from build123d import *

# Parameters (mm, degrees)
SKETCH1_W           = 19.05
SKETCH1_H           = 19.05
SKETCH1_W_2         = 14.2875
SKETCH1_H_2         = 14.2875
BOSS_EXTRUDE1_DEPTH = 25.4
CUT_EXTRUDE1_REACH  = 21.05
SKETCH2_R           = 3.175
SKETCH3_R           = 4
BOSS_EXTRUDE2_DEPTH = 31.75
FILLET1_R           = 2.54


with BuildPart() as part:
    # Sketch1 → Boss-Extrude1 (new body)
    with BuildSketch(Plane(origin=(0, 0, 0), x_dir=(1, 0, 0), z_dir=(0, 1, 0))):
        with Locations((9.525, 9.525)):
            Rectangle(SKETCH1_W, SKETCH1_H)
        with Locations((9.525, 9.525)):
            Rectangle(SKETCH1_W_2, SKETCH1_H_2, mode=Mode.SUBTRACT)
    extrude(amount=BOSS_EXTRUDE1_DEPTH)

    # Sketch2 → Cut-Extrude1 (cut, up to next)
    with BuildSketch(Plane.XY, mode=Mode.PRIVATE) as cut_extrude1_sk1:
        with Locations((9.525, 12.7)):
            Circle(SKETCH2_R)
    cut_extrude1_tool1 = extrude(cut_extrude1_sk1.sketch, amount=-CUT_EXTRUDE1_REACH, mode=Mode.PRIVATE) & part.part
    add(cut_extrude1_tool1.solids().sort_by_distance((9.525, 12.7, 0))[0], mode=Mode.SUBTRACT)

    # Sketch3 → Boss-Extrude2 (add)
    with BuildSketch(Plane(origin=(19.05, 0, 0), x_dir=(0, 0, -1), z_dir=(1, 0, 0))):
        with Locations((9.525, 12.7)):
            Circle(SKETCH3_R)
    extrude(amount=BOSS_EXTRUDE2_DEPTH)

    # Fillet1
    fillet1_edges = [part.edges().sort_by_distance(p)[0] for p in [
        (2.38125, 12.7, -16.66875),
        (2.38125, 12.7, -2.38125),
        (16.66875, 12.7, -2.38125),
        (16.66875, 12.7, -16.66875),
        (0, 12.7, -19.05),
        (19.05, 12.7, -19.05),
        (19.05, 12.7, 0),
        (0, 12.7, 0),
    ]]
    fillet(fillet1_edges, radius=FILLET1_R)


solid = part.part
Input: part model. Units: mm. Frame: model coordinates. A direction names the side the tool comes from. Give positions to 0.01 mm unless a question says otherwise; leave off trailing zeros. Order: outer loops, then holes, each group sorted by start corner. A loop starts at its lowest first (then second) coordinate and runs counter-clockwise, first axis right, second up. Notation, with made-up numbers: (9.5, -9.5) - (47.5, -9.5) arc R16 ccw to (47.5, 18.5) - close; hole circle Ø5 at (29.25, 18). An arc over 180 degrees is marked (long way). Write each question's results on one line, items separated by ' | '.
Item 1: Section C-C (y = 12.7). Return loops of the section in (x, z) (3 decimals).
A:
outline: (0, -16.51) arc R2.54 ccw to (2.54, -19.05) - (16.51, -19.05) arc R2.54 ccw to (19.05, -16.51) - (19.05, -13.525) - (50.8, -13.525) - (50.8, -5.525) - (19.05, -5.525) - (19.05, -2.54) arc R2.54 ccw to (16.51, 0) - (12.7, 0) - (12.7, -2.381) - (14.129, -2.381) arc R2.54 cw to (16.669, -4.921) - (16.669, -14.129) arc R2.54 cw to (14.129, -16.669) - (4.921, -16.669) arc R2.54 cw to (2.381, -14.129) - (2.381, -4.921) arc R2.54 cw to (4.921, -2.381) - (6.35, -2.381) - (6.35, 0) - (2.54, 0) arc R2.54 ccw to (0, -2.54) - close
Item 2: Contact query for flat-ended pins moving along their axis: pin 1 Ø4 at (x, z) = (27.5, -10.5) entering from +Y; pin 2 Ø12 at (x, y) = (45.5, 22) entering from +Z; pin 3 Ø2 at (y, z) = (7, -4) entering from +X. Output: stop coordinate, or through.
A:
pin 1: stops at y = 16.7 | pin 2: stops at z = -7.26 | pin 3: stops at x = 19.05
Item 3: Section D-D (x = 30). Return loops of the section in (y, z) (3 decimals), and give its area (3 significant figures).
A:
outline: circle Ø8 at (12.7, -9.525) | area: 50.3 mm^2
Item 4: Access query for faces 5 (the cylindrical face through (34.7, 9.15, -11.37)), 6 (the cylindrical face through (18.286, 12.878, -0.724)), 7 (the cylindrical face through (3.145, 12.878, -3.106)). Directions: +Z, -Z, +X, -X, +Y, -Y. A direction counts if a zero-diameter tool reaches every point of the face in a straight line with its end or side. Return the directions, or none.
A:
face 5: +X | face 6: +Z, +X, +Y, -Y | face 7: +Y, -Y
Item 5: Section B-B (z = -15.5). Return loops of the section in (x, y).
A:
outline: (0, 0) - (2.78, 0) - (2.78, 25.4) - (0, 25.4) - close; (16.27, 0) - (19.05, 0) - (19.05, 25.4) - (16.27, 25.4) - close
Item 6: Section A-A (y = 3.75). Return loops of the section in (x, z), and give its area (3 significant figures).
A:
outline: (0, -16.51) arc R2.54 ccw to (2.54, -19.05) - (16.51, -19.05) arc R2.54 ccw to (19.05, -16.51) - (19.05, -2.54) arc R2.54 ccw to (16.51, 0) - (2.54, 0) arc R2.54 ccw to (0, -2.54) - close; hole (2.38, -14.13) arc R2.54 ccw to (4.92, -16.67) - (14.13, -16.67) arc R2.54 ccw to (16.67, -14.13) - (16.67, -4.92) arc R2.54 ccw to (14.13, -2.38) - (4.92, -2.38) arc R2.54 ccw to (2.38, -4.92) - close | area: 159 mm^2
Item 7: Material intervals for line 1 along X through (y, z) = (14.25, -7.75); line 2 along Z through (x, y) = (10.5, 9.25); line 3 along X through (y, z) = (1.5, -9.75), sorted ascending.
A:
line 1: x = 0 to 2.38, 16.67 to 50.8 | line 2: z = -19.05 to -16.67, -2.38 to 0 | line 3: x = 0 to 2.38, 16.67 to 19.05
Item 8: Draft query along X for faces 1 (the flat face through (50.8, 13, -9)), 2 (the cylindrical face through (0.724, 12.878, -18.286)), 3 (the flat face through (9, 13, -16.669)), 4 (the flat face through (9, 0, -18)). Return one class per face: released by +X, released by -X, zero draft, split by the parting line, or undercut.
A:
face 1: released by +X | face 2: released by -X | face 3: undercut | face 4: zero draft
